from build123d import *

# Parameters (mm, degrees)
BOSS_EXTRUDE4_DEPTH = 5
SKETCH7_R           = 3
CUT_EXTRUDE4_DEPTH  = 2
SKETCH8_W           = 70
SKETCH8_H           = 70
BOSS_EXTRUDE5_DEPTH = 30
MIRROR2_START       = 5
MIRROR2_OUTLINE_W   = 70
MIRROR2_OUTLINE_H   = 70
MIRROR2_DEPTH       = 30
MIRROR2_2_OUTLINE_R = 3
MIRROR2_2_DEPTH     = 5
MIRROR2_START_2     = 2
MIRROR2_3_OUTLINE_R = 3
MIRROR2_3_DEPTH     = 3
FILLET1_R           = 10
CUT_EXTRUDE5_DEPTH  = 30
BOSS_EXTRUDE6_DEPTH = 2.5
CHAMFER1_SIZE       = 1.25


# Read off the part's stored shape, not the designer's step: Mirror2
with BuildPart() as part:
    # Sketch5 → Boss-Extrude4 (new body)
    with BuildSketch(Plane(origin=(0, 0, 0), x_dir=(1, 0, 0), z_dir=(0, 1, 0))):
        with BuildLine():
            Line((-22.5, -32.5), (22.5, -32.5))
            ThreePointArc((22.5, -32.5), (29.571067812, -29.571067812), (32.5, -22.5))
            Line((32.5, -22.5), (32.5, 22.5))
            ThreePointArc((32.5, 22.5), (29.571067812, 29.571067812), (22.5, 32.5))
            Line((22.5, 32.5), (-22.5, 32.5))
            ThreePointArc((-22.5, 32.5), (-29.571067812, 29.571067812), (-32.5, 22.5))
            Line((-32.5, 22.5), (-32.5, -22.5))
            ThreePointArc((-32.5, -22.5), (-29.571067812, -29.571067812), (-22.5, -32.5))
        make_face()
    extrude(amount=BOSS_EXTRUDE4_DEPTH)

    # Sketch7 → Cut-Extrude4 (cut)
    with BuildSketch(Plane.XZ):
        with Locations(Location((-26.035533906, 26.035533906, 0), (0, 0, 270))):
            Circle(SKETCH7_R)
        with Locations(Location((26.036533906, 26.036533906, 0), (0, 0, 270))):
            Circle(SKETCH7_R)
        with Locations(Location((26.037533906, -26.035533906, 0), (0, 0, 270))):
            Circle(SKETCH7_R)
        with Locations(Location((-26.034533906, -26.036533906, 0), (0, 0, 270))):
            Circle(SKETCH7_R)
    extrude(amount=-CUT_EXTRUDE4_DEPTH, mode=Mode.SUBTRACT)

    # Sketch8 → Boss-Extrude5 (add)
    with BuildSketch(Plane(origin=(0, 5, 0), x_dir=(1, 0, 0), z_dir=(0, 1, 0))):
        Rectangle(SKETCH8_W, SKETCH8_H)
    extrude(amount=BOSS_EXTRUDE5_DEPTH)

    # Mirror2 outline → Mirror2 (add)
    with BuildSketch(Plane(origin=(0, 0, 0), x_dir=(1, 0, 0), z_dir=(0, 1, 0)).offset(MIRROR2_START)):
        with Locations((0, -70)):
            Rectangle(MIRROR2_OUTLINE_W, MIRROR2_OUTLINE_H)
        with Locations((0, 70)):
            Rectangle(MIRROR2_OUTLINE_W, MIRROR2_OUTLINE_H)
    extrude(amount=MIRROR2_DEPTH)

    # Mirror2 2 outline → Mirror2 2 (add)
    # profile 1 of 2: a face of its own
    with BuildSketch(Plane(origin=(0, 0, 0), x_dir=(1, 0, 0), z_dir=(0, 1, 0))):
        with BuildLine():
            Line((32.5, -92.5), (32.5, -47.5))
            ThreePointArc((32.5, -47.5), (29.571067812, -40.428932188), (22.5, -37.5))
            Line((22.5, -37.5), (-22.5, -37.5))
            ThreePointArc((-22.5, -37.5), (-29.571067812, -40.428932188), (-32.5, -47.5))
            Line((-32.5, -47.5), (-32.5, -92.5))
            ThreePointArc((-32.5, -92.5), (-29.571067812, -99.571067812), (-22.5, -102.5))
            Line((-22.5, -102.5), (22.5, -102.5))
            ThreePointArc((22.5, -102.5), (29.571067812, -99.571067812), (32.5, -92.5))
        make_face()
        with Locations((-26.034533906, -96.036533906)):
            Circle(MIRROR2_2_OUTLINE_R, mode=Mode.SUBTRACT)
        with Locations((-26.035533906, -43.964466094)):
            Circle(MIRROR2_2_OUTLINE_R, mode=Mode.SUBTRACT)
        with Locations((26.037533906, -96.035533906)):
            Circle(MIRROR2_2_OUTLINE_R, mode=Mode.SUBTRACT)
        with Locations((26.036533906, -43.963466094)):
            Circle(MIRROR2_2_OUTLINE_R, mode=Mode.SUBTRACT)
    # profile 2 of 2: a face of its own
    with BuildSketch(Plane(origin=(0, 0, 0), x_dir=(1, 0, 0), z_dir=(0, 1, 0))):
        with BuildLine():
            Line((32.5, 47.5), (32.5, 92.5))
            ThreePointArc((32.5, 92.5), (29.571067812, 99.571067812), (22.5, 102.5))
            Line((22.5, 102.5), (-22.5, 102.5))
            ThreePointArc((-22.5, 102.5), (-29.571067812, 99.571067812), (-32.5, 92.5))
            Line((-32.5, 92.5), (-32.5, 47.5))
            ThreePointArc((-32.5, 47.5), (-29.571067812, 40.428932188), (-22.5, 37.5))
            Line((-22.5, 37.5), (22.5, 37.5))
            ThreePointArc((22.5, 37.5), (29.571067812, 40.428932188), (32.5, 47.5))
        make_face()
        with Locations((-26.034533906, 43.963466094)):
            Circle(MIRROR2_2_OUTLINE_R, mode=Mode.SUBTRACT)
        with Locations((-26.035533906, 96.035533906)):
            Circle(MIRROR2_2_OUTLINE_R, mode=Mode.SUBTRACT)
        with Locations((26.037533906, 43.964466094)):
            Circle(MIRROR2_2_OUTLINE_R, mode=Mode.SUBTRACT)
        with Locations((26.036533906, 96.036533906)):
            Circle(MIRROR2_2_OUTLINE_R, mode=Mode.SUBTRACT)
    extrude(amount=MIRROR2_2_DEPTH)

    # Mirror2 3 outline → Mirror2 3 (add)
    with BuildSketch(Plane(origin=(0, 0, 0), x_dir=(1, 0, 0), z_dir=(0, 1, 0)).offset(MIRROR2_START_2)):
        with Locations((-26.035533906, -43.964466094)):
            Circle(MIRROR2_3_OUTLINE_R)
        with Locations((26.036533906, -43.963466094)):
            Circle(MIRROR2_3_OUTLINE_R)
        with Locations((26.037533906, -96.035533906)):
            Circle(MIRROR2_3_OUTLINE_R)
        with Locations((-26.034533906, -96.036533906)):
            Circle(MIRROR2_3_OUTLINE_R)
        with Locations((-26.035533906, 96.035533906)):
            Circle(MIRROR2_3_OUTLINE_R)
        with Locations((26.036533906, 96.036533906)):
            Circle(MIRROR2_3_OUTLINE_R)
        with Locations((26.037533906, 43.964466094)):
            Circle(MIRROR2_3_OUTLINE_R)
        with Locations((-26.034533906, 43.963466094)):
            Circle(MIRROR2_3_OUTLINE_R)
    extrude(amount=MIRROR2_3_DEPTH)

    # Fillet1
    fillet1_edges = [part.edges().sort_by_distance(p)[0] for p in [
        (35, 20, 105),
        (-35, 20, 105),
        (-35, 20, -105),
        (35, 20, -105),
    ]]
    fillet(fillet1_edges, radius=FILLET1_R)

    # Sketch9 → Cut-Extrude5 (cut)
    with BuildSketch(Plane(origin=(0, 35, 0), x_dir=(1, 0, 0), z_dir=(0, 1, 0))):
        with BuildLine():
            Line((-32.5, 95), (-32.5, -95))
            ThreePointArc((-32.5, -95), (-30.303300859, -100.303300859), (-25, -102.5))
            Line((-25, -102.5), (25, -102.5))
            ThreePointArc((25, -102.5), (30.303300859, -100.303300859), (32.5, -95))
            Line((32.5, -95), (32.5, 95))
            ThreePointArc((32.5, 95), (30.303300859, 100.303300859), (25, 102.5))
            Line((25, 102.5), (-25, 102.5))
            ThreePointArc((-25, 102.5), (-30.303300859, 100.303300859), (-32.5, 95))
        make_face()
    extrude(amount=-CUT_EXTRUDE5_DEPTH, mode=Mode.SUBTRACT)


with BuildPart() as cut_extrude5_piece_1:
    # of the separate pieces the step leaves, piece 1, a body of its own (cut_extrude5_pieces)
    add(part.part.solids().sort_by_distance((35, 5, 95))[0])



with BuildPart() as cut_extrude5_piece_2:
    # of the separate pieces the step leaves, piece 2, a body of its own (cut_extrude5_pieces)
    add(part.part.solids().sort_by_distance((32.5, 0, 92.5))[0])


with BuildPart() as cut_extrude5_piece_3:
    # of the separate pieces the step leaves, piece 3, a body of its own (cut_extrude5_pieces)
    add(part.part.solids().sort_by_distance((32.5, 0, -47.5))[0])


with BuildPart() as cut_extrude5_piece_4:
    # of the separate pieces the step leaves, piece 4, a body of its own (cut_extrude5_pieces)
    add(part.part.solids().sort_by_distance((32.5, 0, 22.5))[0])


with BuildPart() as cut_extrude5_piece_1_1:
    add(cut_extrude5_piece_1.part)

    add(cut_extrude5_piece_2.part)  # Boss-Extrude6 merges Cut-Extrude5 piece 2

    add(cut_extrude5_piece_3.part)  # Boss-Extrude6 merges Cut-Extrude5 piece 3

    add(cut_extrude5_piece_4.part)  # Boss-Extrude6 merges Cut-Extrude5 piece 4
    # Sketch10 → Boss-Extrude6 (add)
    with BuildSketch(Plane.XZ.offset(-5)):
        with BuildLine():
            Line((25, 105), (-25, 105))
            ThreePointArc((-25, 105), (-32.071067812, 102.071067812), (-35, 95))
            Line((-35, 95), (-35, -95))
            ThreePointArc((-35, -95), (-32.071067812, -102.071067812), (-25, -105))
            Line((-25, -105), (25, -105))
            ThreePointArc((25, -105), (32.071067812, -102.071067812), (35, -95))
            Line((35, -95), (35, 95))
            ThreePointArc((35, 95), (32.071067812, 102.071067812), (25, 105))
        make_face()
    extrude(amount=-BOSS_EXTRUDE6_DEPTH)

    # Chamfer1
    chamfer1_edges = [cut_extrude5_piece_1_1.edges().sort_by_distance(p)[0] for p in [
        (0, 35, 102.5),
        (-32.5, 35, 0),
        (-30.303300859, 35, 100.303300859),
        (30.303300859, 35, 100.303300859),
        (30.303300859, 35, -100.303300859),
        (-30.303300859, 35, -100.303300859),
        (-30.303300859, 7.5, -100.303300859),
        (0, 7.5, 102.5),
        (30.303300859, 7.5, 100.303300859),
        (32.5, 7.5, 0),
        (30.303300859, 7.5, -100.303300859),
        (0, 7.5, -102.5),
        (-32.5, 7.5, 0),
        (-30.303300859, 7.5, 100.303300859),
        (0, 35, -102.5),
        (32.5, 35, 0),
    ]]
    chamfer(chamfer1_edges, length=CHAMFER1_SIZE)


solid = cut_extrude5_piece_1_1.part
The model under review builds one solid part; all positions refer to its coordinate system, in mm. A direction names the side the tool comes from. Round coordinates to 2 decimals unless told otherwise and drop trailing zeros. Loops run counter-clockwise (first coordinate to the right, second up) from the corner with the lowest first, then second, coordinate; pieces in that order, holes last. Notation, with made-up numbers: (41, 76.25) -> (64, 76.25) arc R22 cw to (64, 106.25) -> close; hole circle Ø7 at (84.5, -31). An arc over 180 degrees is marked (long way). Return JSON: item names as keys, results as strings.
(1) Add section C-C on y = 19.5. Write out the cut boundary in (x, z).
Solved:
{"outline": "(-35, -95) arc R10 ccw to (-25, -105) -> (25, -105) arc R10 ccw to (35, -95) -> (35, 95) arc R10 ccw to (25, 105) -> (-25, 105) arc R10 ccw to (-35, 95) -> close; hole (-32.5, -95) arc R7.5 ccw to (-25, -102.5) -> (25, -102.5) arc R7.5 ccw to (32.5, -95) -> (32.5, 95) arc R7.5 ccw to (25, 102.5) -> (-25, 102.5) arc R7.5 ccw to (-32.5, 95) -> close"}
(2) The part is to be moulded in two halves that separate along X. For faces 1 (the flat face through (0, 2, 37.5)), 2 (the cylindrical face through (32.15, 20.21, -101.99)), 3 (the cylindrical face through (30.361, 21.425, -100.245)), 4 (the flat face through (-32.5, 2, 70)), say which applies: released by +X, released by -X, zero draft, split by the parting line, or undercut.
Solved:
{"face 1": "zero draft", "face 2": "released by +X", "face 3": "undercut", "face 4": "released by -X"}
(3) For line 1 (X direction, y = 26, z = -6); line 2 (Z direction, x = 5.5, y = 4); line 3 (Z direction, x = 6, y = 10), list the stretches that pass through material, from the lowest coordinate up.
Solved:
{"line 1": "-35 to -32.5, 32.5 to 35", "line 2": "-102.5 to -37.5, -32.5 to 32.5, 37.5 to 102.5", "line 3": "-105 to -102.5, 102.5 to 105"}
(4) Add section A-A on z = -87.5. Write out the cut boundary in (x, y), plus the area to 4 significant figures.
Solved:
{"outline": "(-35, 5) -> (-32.5, 5) -> (-32.5, 0) -> (32.5, 0) -> (32.5, 5) -> (35, 5) -> (35, 35) -> (33.75, 35) -> (32.5, 33.75) -> (32.5, 8.75) -> (31.25, 7.5) -> (-31.25, 7.5) -> (-32.5, 8.75) -> (-32.5, 33.75) -> (-33.75, 35) -> (-35, 35) -> close", "area": "637.5 mm2"}
(5) Add section B-B on x = -13.5. Write out the cut boundary in (y, z).
Solved:
{"outline": "(0, -102.5) -> (5, -102.5) -> (5, -105) -> (35, -105) -> (35, -103.75) -> (33.75, -102.5) -> (8.75, -102.5) -> (7.5, -101.25) -> (7.5, 101.25) -> (8.75, 102.5) -> (33.75, 102.5) -> (35, 103.75) -> (35, 105) -> (5, 105) -> (5, 102.5) -> (0, 102.5) -> (0, 37.5) -> (5, 37.5) -> (5, 32.5) -> (0, 32.5) -> (0, -32.5) -> (5, -32.5) -> (5, -37.5) -> (0, -37.5) -> close"}
(6) For pin 1 (5 mm diameter, centred on x = 26.04, z = -26.04, fed in from +Y); pin 2 (1.8 mm diameter, centred on x = -26.5, z = -42.5, fed in from -Y); pin 3 (1.5 mm diameter, centred on y = 1.5, z = 79, fed in from +X), all flat-tipped, find the tip position at first contact; note any pin that passes through.
Solved:
{"pin 1": "y = 7.5", "pin 2": "y = 2", "pin 3": "x = 32.5"}
(7) For faces 5 (the flat face through (26, 2, -44)), 6 (the cylindrical face through (-29.65, 2.46, 29.49)), 7 (the conical face through (29.61, 7.84, 99.71)), 8 (the cylindrical face through (29.65, 2.46, -29.49)), list the 3-axis set-ups (+Z, -Z, +X, -X, +Y, -Y) from which the entire face can be reached by the end or side of a thin tool; tool diameter is ignored.
Solved:
{"face 5": "-Y", "face 6": "-X, -Y", "face 7": "+Y", "face 8": "+X, -Y"}
